Study the drawing (mm; zero at the part's minimum x, y, z) and answer. A direction names the side the tool comes from. Coordinates: 2 decimals unless noted, no trailing zeros. Write each loop counter-clockwise with the first axis right and the second up, starting at its lowest first coordinate (ties: lowest second). Pieces come first, ordered by that corner, then holes. Notation, with made-up numbers: (49, -13) -> (104, -13) arc R17 cw to (104, -7) -> close; hole circle Ø11 at (4, -13.5). An arc over 180 degrees is marked (long way). Answer in a Markdown table with one row per item. Add a question column.
Item 1: Which of the six approach directions +Z, -Z, +X, -X, +Y, -Y give full straight-line access (tool end or side, diameter ignored) to the marked faces 1, 2 and 3?
Item 2: Section C-C on x = 54 is taken. Write down the section's boundary in (y, z).
Item 3: Given pin 1 Ø6 at (x, z) = (48, 8) entering from -Y; pin 2 Ø1.5 at (x, y) = (25, 9.5) entering from -Z; pin 3 Ø2 at (x, y) = (36, 3) entering from -Z, each flat-ended and moving along its own axis, determine where each tip first touches the part or whether it passes through.
Item 4: Straight lines are drawn through the part: line 1 (X direction, y = 2.75, z = 8) (1 decimal); line 2 (Y direction, x = 10, z = 6); line 3 (X direction, y = 3, z = 10) (1 decimal). For each, find the intervals that lie inside material, in ascending order. Write a range as from..to.
Item 5: Section B-B on y = 6.5 is taken. Write down the section's boundary in (x, z) (1 decimal), then the cut area to 3 significant figures.
Item 6: Section A-A on z = 6 is taken. Write down the section's boundary in (x, y) (1 decimal), then the cut area to 3 significant figures.
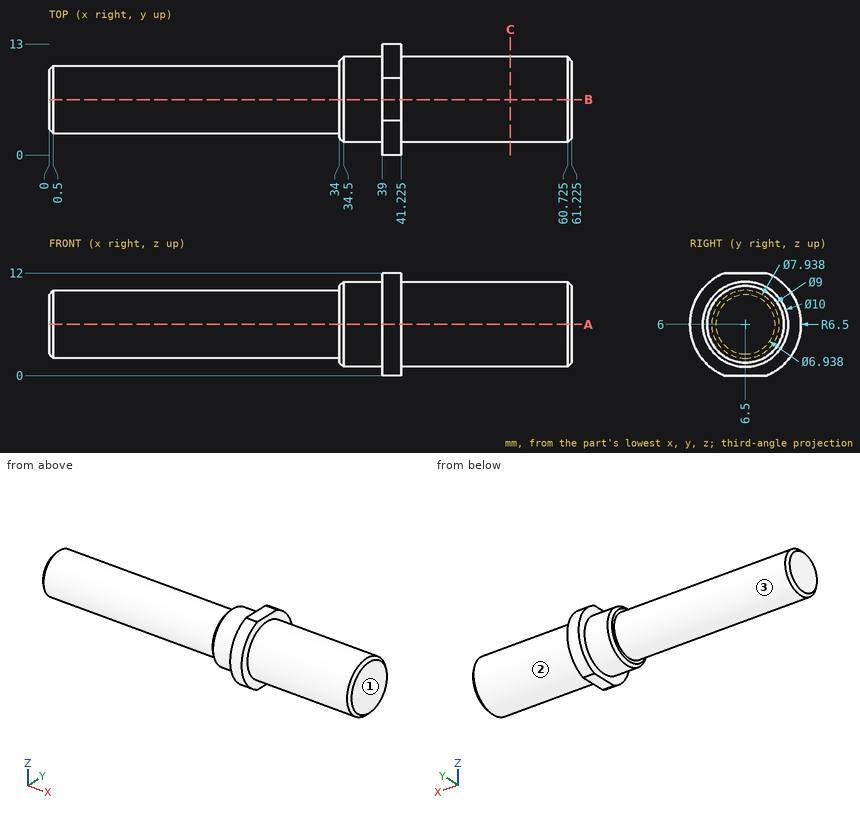
Results below:
| question | item | result |
|---|---|---|
| 1 | face 1 | +Z, -Z, +X, +Y, -Y |
| 1 | face 2 | +X |
| 1 | face 3 | -X |
| 2 | outline | circle Ø10 at (6.5, 6) |
| 3 | pin 1 | stops at y = 1.5 |
| 3 | pin 2 | stops at z = 2.73 |
| 3 | pin 3 | stops at z = 1.67 |
| 4 | line 1 | x = 34..61.2 |
| 4 | line 2 | y = 2.53..10.47 |
| 4 | line 3 | x = 39..41.2 |
| 5 | outline | (0, 2.5) -> (0.5, 2) -> (34, 2) -> (34, 1.5) -> (34.5, 1) -> (39, 1) -> (39, 0) -> (41.2, 0) -> (41.2, 1) -> (60.7, 1) -> (61.2, 1.5) -> (61.2, 10.5) -> (60.7, 11) -> (41.2, 11) -> (41.2, 12) -> (39, 12) -> (39, 11) -> (34.5, 11) -> (34, 10.5) -> (34, 10) -> (0.5, 10) -> (0, 9.5) -> close |
| 5 | area | 546 mm2 |
| 6 | outline | (0, 3) -> (0.5, 2.5) -> (34, 2.5) -> (34, 2) -> (34.5, 1.5) -> (39, 1.5) -> (39, 0) -> (41.2, 0) -> (41.2, 1.5) -> (60.7, 1.5) -> (61.2, 2) -> (61.2, 11) -> (60.7, 11.5) -> (41.2, 11.5) -> (41.2, 13) -> (39, 13) -> (39, 11.5) -> (34.5, 11.5) -> (34, 11) -> (34, 10.5) -> (0.5, 10.5) -> (0, 10) -> close |
| 6 | area | 548 mm2 |
